Geometry: final body of the model. Coordinates: model frame, mm. A direction names the side the tool comes from. Give positions to 0.01 mm unless a question says otherwise; leave off trailing zeros. Loops run counter-clockwise (first coordinate to the right, second up) from the corner with the lowest first, then second, coordinate; pieces in that order, holes last.
1. Draft query along Y for faces 4 (the face through (13, 47.339, 63)), 5 (the face through (25.4, 38, 50)). Return one class per face: +Y half, -Y half, draft (parallel to the pull), parting line (faces both ways), or undercut.
2. Access query for faces 1 (the face through (17, 67.945, 16)), 2 (the face through (3.287, 36.586, 13.177)), 3 (the face through (5.08, 49, 64)). Directions: +Z, -Z, +X, -X, +Y, -Y. A direction counts if a zero-diameter tool reaches every point of the face in a straight line with its end or side. Return the directions, or none.
3. Section A-A, the plane z = 12.7. Output: boundary loops of the cut face in (x, y) (1 decimal).
4. Section B-B, the plane z = 71.5. State how many separate pieces and enclosed holes the cut face has, then the cut area to 3 significant figures.
5. Material intervals for line 1 along Z through (x, y) = (3.25, 38.1); line 2 along X through (y, z) = (68.5, 63.5); line 3 along Z through (x, y) = (18.5, 47) (3 decimals), sorted ascending.
6. First-contact query: P1, Ø2, axis at x = 11, y = 33.5, coming from the +Z side. Flat tip, straight axial feed; report the tip coordinate or a pass-through.
from build123d import *

# Parameters (mm, degrees)
F0_W      = 25.4
F0_H      = 76.2
F1_DEPTH  = 101.6
F2_W      = 15.24
F2_H      = 66.04
F3_DEPTH  = 76.2
F6_START  = -3.175
F5_W      = 3.175
F5_H      = 59.69
F6_DEPTH  = 12.065
F4_R      = 1.5875
F7_DEPTH  = 6.6675
F8_R      = 1.5875
F9_DEPTH  = 6.6675
F10_W     = 1.5875
F10_H     = 1.5875
F11_DEPTH = 3.175
F12_W     = 1.5875
F12_H     = 1.5875
F13_DEPTH = 3.175
F14_W     = 15.24
F14_H     = 0.396875
F15_DEPTH = 76.2


with BuildPart() as f1:
    # F0 (on Top) → F1 (new body)
    with BuildSketch(Plane.XY):
        with Locations((12.7, 38.1)):
            Rectangle(F0_W, F0_H)
    extrude(amount=F1_DEPTH)

    # F2 (on face) → F3 (cut)
    with BuildSketch(Plane.XY.offset(101.6)):
        with Locations((12.7, 38.1)):
            Rectangle(F2_W, F2_H)
    extrude(amount=-F3_DEPTH, mode=Mode.SUBTRACT)

    # F5 (on face) → F6 (cut)
    with BuildSketch(Plane.XY.offset(25.4).offset(F6_START)):
        with Locations((17.145, 38.1)):
            Rectangle(F5_W, F5_H)
        with Locations((8.255, 38.1)):
            Rectangle(F5_W, F5_H)
    extrude(amount=-F6_DEPTH, mode=Mode.SUBTRACT)

    # F4 (on face) → F7 (cut, through all)
    with BuildSketch(Plane.YZ.offset(25.4)):
        with Locations((38.1, 12.7)):
            Circle(F4_R)
    extrude(amount=-F7_DEPTH, mode=Mode.SUBTRACT)

    # F8 (on face) → F9 (cut, through all)
    with BuildSketch(Plane(origin=(0, 0, 0), x_dir=(0, -1, 0), z_dir=(-1, 0, 0))):
        with Locations((-38.1, 12.7)):
            Circle(F8_R)
    extrude(amount=-F9_DEPTH, mode=Mode.SUBTRACT)

    # F10 (on face) → F11 (cut, through all)
    with BuildSketch(Plane.XY.offset(25.4)):
        with Locations((8.255, 64.9995461683)):
            Rectangle(F10_W, F10_H)
        with Locations((8.255, 58.6495461683)):
            Rectangle(F10_W, F10_H)
        with Locations((8.255, 52.2995461683)):
            Rectangle(F10_W, F10_H)
        with Locations((8.255, 45.9495461683)):
            Rectangle(F10_W, F10_H)
        with Locations((8.255, 39.5995461683)):
            Rectangle(F10_W, F10_H)
        with Locations((8.255, 33.2495461683)):
            Rectangle(F10_W, F10_H)
        with Locations((8.255, 26.8995461683)):
            Rectangle(F10_W, F10_H)
        with Locations((8.255, 20.5495461683)):
            Rectangle(F10_W, F10_H)
        with Locations((8.255, 14.1995461683)):
            Rectangle(F10_W, F10_H)
    extrude(amount=-F11_DEPTH, mode=Mode.SUBTRACT)

    # F12 (on face) → F13 (cut, through all)
    with BuildSketch(Plane.XY.offset(25.4)):
        with Locations((17.145, 61.8245461683)):
            Rectangle(F12_W, F12_H)
        with Locations((17.145, 55.4745461683)):
            Rectangle(F12_W, F12_H)
        with Locations((17.145, 49.1245461683)):
            Rectangle(F12_W, F12_H)
        with Locations((17.145, 42.7745461683)):
            Rectangle(F12_W, F12_H)
        with Locations((17.145, 36.4245461683)):
            Rectangle(F12_W, F12_H)
        with Locations((17.145, 30.0745461683)):
            Rectangle(F12_W, F12_H)
        with Locations((17.145, 23.7245461683)):
            Rectangle(F12_W, F12_H)
        with Locations((17.145, 17.3745461683)):
            Rectangle(F12_W, F12_H)
        with Locations((17.145, 11.0245461683)):
            Rectangle(F12_W, F12_H)
    extrude(amount=-F13_DEPTH, mode=Mode.SUBTRACT)

    # F14 (on face) → F15 (join, through all)
    with BuildSketch(Plane.XY.offset(25.4)):
        with Locations((12.7, 63.4120461683)):
            Rectangle(F14_W, F14_H)
        with Locations((12.7, 60.2370461683)):
            Rectangle(F14_W, F14_H)
        with Locations((12.7, 57.0620461683)):
            Rectangle(F14_W, F14_H)
        with Locations((12.7, 53.8870461683)):
            Rectangle(F14_W, F14_H)
        with Locations((12.7, 50.7120461683)):
            Rectangle(F14_W, F14_H)
        with Locations((12.7, 47.5370461683)):
            Rectangle(F14_W, F14_H)
        with Locations((12.7, 44.3620461683)):
            Rectangle(F14_W, F14_H)
        with Locations((12.7, 41.1870461683)):
            Rectangle(F14_W, F14_H)
        with Locations((12.7, 38.0120461683)):
            Rectangle(F14_W, F14_H)
        with Locations((12.7, 34.8370461683)):
            Rectangle(F14_W, F14_H)
        with Locations((12.7, 31.6620461683)):
            Rectangle(F14_W, F14_H)
        with Locations((12.7, 28.4870461683)):
            Rectangle(F14_W, F14_H)
        with Locations((12.7, 25.3120461683)):
            Rectangle(F14_W, F14_H)
        with Locations((12.7, 22.1370461683)):
            Rectangle(F14_W, F14_H)
        with Locations((12.7, 18.9620461683)):
            Rectangle(F14_W, F14_H)
        with Locations((12.7, 15.7870461683)):
            Rectangle(F14_W, F14_H)
        with Locations((12.7, 12.6120461683)):
            Rectangle(F14_W, F14_H)
    extrude(amount=F15_DEPTH)


solid = f1.part
Answers below:
1. face 4: undercut
1. face 5: draft
2. face 1: none
2. face 2: -X
2. face 3: +Z
3. outline: (0, 0) - (25.4, 0) - (25.4, 36.5) - (18.7, 36.5) - (18.7, 8.3) - (15.6, 8.3) - (15.6, 67.9) - (18.7, 67.9) - (18.7, 39.7) - (25.4, 39.7) - (25.4, 76.2) - (0, 76.2) - (0, 39.7) - (6.7, 39.7) - (6.7, 67.9) - (9.8, 67.9) - (9.8, 8.3) - (6.7, 8.3) - (6.7, 36.5) - (0, 36.5) - close
4. separate pieces: 1
4. enclosed holes: 18
4. area: 1,030 mm2
5. line 1: z = 0 to 11.11, 14.29 to 101.6
5. line 2: x = 0 to 5.08, 20.32 to 25.4
5. line 3: z = 0 to 10.16, 22.225 to 25.4
6. P1: stops at z = 25.4
